Here's how the part is built. I have some questions about the finished solid (model axes, mm). Round coordinates to 2 decimals unless told otherwise and drop trailing zeros. Use one line per item in the form item = value. Start each with the question number.
Item 1: If I drill on L1, parallel to Z at x = 7.5, y = -4; L2, parallel to Y at x = -3, z = 6.5; L3, parallel to Z at x = -5.5, y = -7, over which ranges is the centre line in solid material (lowest first)? Write a range as [from, to].
Item 2: Thinking about a two-plate mould opening in Z: for faces 1 (the face through (0, 0, 0)), 2 (the face through (-2.175, -9.794, 1.288)), 3 (the face through (2.04, -0.06, 32.55)), 4 (the face through (-0.08, -0.34, 37.11)), which applies, released by +Z, released by -Z, zero draft, split by the parting line, or undercut?
Item 3: I'm going to push flat-ended pins straight in: pin 1 Ø1 at (y, z) = (2.5, 20) entering from -X; pin 2 Ø4 at (x, y) = (-4, -2.5) entering from +Z; pin 3 Ø5 at (y, z) = (3, 27.5) entering from -X. Where does each tip first touch, or does it pass through?
```python
from build123d import *

# Parameters (mm, degrees)
F2_DEPTH = 25.4
F3_DEPTH = 25.4


with BuildPart() as f1:
    # F0 (on Front) → F1 (revolve)
    with BuildSketch(Plane.XZ):
        Polygon((0, 2.54), (0, 0), (10.033, 0), (10.033, 2.54), (9.4861555845, 2.54), align=None)
        with BuildLine():
            Line((0, 37.1824353933), (0, 2.54))
            Line((0, 2.54), (9.4861555845, 2.54))
            add(Edge.make_bspline(
                [(9.4861555845, 2.54), (9.8453891211, 4.4276976498), (5.9179255985, 5.2618132952), (5.1336004733, 7.762343265), (4.2204660289, 11.2245860249), (3.9645507932, 12.6038566232)],
                knots=[0, 0, 0, 0, 0.3490450724, 0.624870565, 1, 1, 1, 1], degree=3))
            Line((3.9645507932, 12.6038566232), (3.5626941826, 12.6038566232))
            add(Edge.make_bspline(
                [(3.5626941826, 12.6038566232), (3.2031516008, 13.3255932383), (2.4760706241, 16.8640443681), (2.3654149475, 19.4231070959), (2.8490578857, 23.2332946699), (3.0645283405, 23.775851354)],
                knots=[0, 0, 0, 0, 0.3450697936, 0.657036582, 1, 1, 1, 1], degree=3))
            Line((3.0645283405, 23.775851354), (3.9743119851, 24.5918147266))
            Line((3.9743119851, 24.5918147266), (3.0645283405, 25.425276343))
            Line((3.0645283405, 25.425276343), (3.0645283405, 25.5275927484))
            add(Edge.make_bspline(
                [(3.0645283405, 25.5275927484), (3.3999102429, 28.2161597708), (4.9036466919, 31.6129373063), (4.7012289547, 32.4872237799), (3.7060201327, 33.5572204547), (2.9138410483, 34.2374070059), (2.8228225087, 34.3145662132)],
                knots=[0, 0, 0, 0, 0.3715523633, 0.4947830291, 0.7141040095, 0.7421667067, 0.7421667067, 0.7421667067, 0.7421667067], degree=3))
            Line((2.8228225087, 34.3145662132), (1.5574188822, 31.4649180467))
            Line((1.5574188822, 31.4649180467), (1.1711250779, 31.6364541636))
            Line((1.1711250779, 31.6364541636), (2.4859273687, 34.597346529))
            add(Edge.make_bspline(
                [(2.4859273687, 34.597346529), (1.7439141747, 35.2174579169), (0.9664492324, 35.8714870687), (0.401673026, 36.7812261591)],
                knots=[0.7763528136, 0.7763528136, 0.7763528136, 0.7763528136, 1, 1, 1, 1], degree=3))
            Line((0.401673026, 36.7812261591), (0.3172948102, 37.3098490119))
            ThreePointArc((0.3172948102, 37.3098490119), (0.1709606876, 37.2154787565), (0, 37.1824353933))
        make_face()
        with BuildLine():
            Line((0, 38.1), (0, 37.1824353933))
            ThreePointArc((0, 37.1824353933), (0.1709606876, 37.2154787565), (0.3172948102, 37.3098490119))
            ThreePointArc((0.3172948102, 37.3098490119), (0.4219303531, 37.4610622666), (0.4587823033, 37.6412176967))
            ThreePointArc((0.4587823033, 37.6412176967), (0.3244080778, 37.9656257744), (0, 38.1))
        make_face()
        with BuildLine():
            add(Edge.make_bspline(
                [(2.8228225087, 34.3145662132), (2.7119433048, 34.4085619146), (2.5993495081, 34.5025579715), (2.4859273687, 34.597346529)],
                knots=[0.7421667067, 0.7421667067, 0.7421667067, 0.7421667067, 0.7763528136, 0.7763528136, 0.7763528136, 0.7763528136], degree=3))
            Line((2.4859273687, 34.597346529), (1.1711250779, 31.6364541636))
            Line((1.1711250779, 31.6364541636), (1.5574188822, 31.4649180467))
            Line((1.5574188822, 31.4649180467), (2.8228225087, 34.3145662132))
        make_face()
    revolve(axis=Axis((0, 0, 19.05), (0, 0, 1)))

    # F0 (on Front) → F2 (cut)
    with BuildSketch(Plane.XZ):
        with BuildLine():
            Line((3.5590358397, 37.0139522053), (2.4859273687, 34.597346529))
            add(Edge.make_bspline(
                [(2.8228225087, 34.3145662132), (2.7119433048, 34.4085619146), (2.5993495081, 34.5025579715), (2.4859273687, 34.597346529)],
                knots=[0.7421667067, 0.7421667067, 0.7421667067, 0.7421667067, 0.7763528136, 0.7763528136, 0.7763528136, 0.7763528136], degree=3))
            Line((2.8228225087, 34.3145662132), (3.9516790885, 36.8567148328))
            Line((3.9516790885, 36.8567148328), (3.5590358397, 37.0139522053))
        make_face()
        with BuildLine():
            add(Edge.make_bspline(
                [(2.8228225087, 34.3145662132), (2.7119433048, 34.4085619146), (2.5993495081, 34.5025579715), (2.4859273687, 34.597346529)],
                knots=[0.7421667067, 0.7421667067, 0.7421667067, 0.7421667067, 0.7763528136, 0.7763528136, 0.7763528136, 0.7763528136], degree=3))
            Line((2.4859273687, 34.597346529), (1.1711250779, 31.6364541636))
            Line((1.1711250779, 31.6364541636), (1.5574188822, 31.4649180467))
            Line((1.5574188822, 31.4649180467), (2.8228225087, 34.3145662132))
        make_face()
    extrude(amount=-F2_DEPTH, mode=Mode.SUBTRACT)

    # F3 (cut): a face of the model
    f3_faces = [f1.faces().sort_by_distance(p)[0] for p in [
        (2.0082250792, 0, 33.0041671759),
    ]]
    extrude(f3_faces, amount=-F3_DEPTH, mode=Mode.SUBTRACT)


solid = f1.part
```
Values found:
q1.L1 = [0, 4.55]
q1.L2 = [-4.77, 4.77]
q1.L3 = [0, 4.25]
q2.face_1 = released by -Z
q2.face_2 = zero draft
q2.face_3 = undercut
q2.face_4 = undercut
q3.pin_1 = -1.52
q3.pin_2 = 34.4
q3.pin_3 = -3.75
